from build123d import *

# Parameters (mm, degrees)
SKETCH1_R                    = 19.05
BOSS_EXTRUDE1_DEPTH          = 272.1102
SKETCH2_R                    = 12.7
CUT_EXTRUDE1_DEPTH           = 273.1102
F_1_1_4_7_TAPPED_HOLE1_D     = 28.17876
F_1_1_4_7_TAPPED_HOLE1_DEPTH = 49.022
F_1_1_4_7_TAPPED_HOLE1_TIP   = 8.465753589
F_1_1_4_7_TAPPED_HOLE2_D     = 28.17876
F_1_1_4_7_TAPPED_HOLE2_DEPTH = 49.022
F_1_1_4_7_TAPPED_HOLE2_TIP   = 8.465753589


with BuildPart() as part:
    # Sketch1 → Boss-Extrude1 (new body)
    with BuildSketch(Plane(origin=(0, 0, 0), x_dir=(1, 0, 0), z_dir=(0, 1, 0))):
        Circle(SKETCH1_R)
    extrude(amount=BOSS_EXTRUDE1_DEPTH)

    # Sketch2 → Cut-Extrude1 (cut, through all)
    with BuildSketch(Plane(origin=(0, 272.1102, 0), x_dir=(1, 0, 0), z_dir=(0, 1, 0))):
        Circle(SKETCH2_R)
    extrude(amount=-CUT_EXTRUDE1_DEPTH, mode=Mode.SUBTRACT)

    # 1-1/4-7 Tapped Hole1
    with Locations(Plane(origin=(0, 272.1102, 0), x_dir=(1, 0, 0), z_dir=(0, 1, 0))):
        with Locations((0, 0)):
            Hole(F_1_1_4_7_TAPPED_HOLE1_D / 2, depth=F_1_1_4_7_TAPPED_HOLE1_DEPTH)
            with Locations((0, 0, -(F_1_1_4_7_TAPPED_HOLE1_DEPTH + F_1_1_4_7_TAPPED_HOLE1_TIP / 2))):  # 118° drill point
                Cone(0, F_1_1_4_7_TAPPED_HOLE1_D / 2, F_1_1_4_7_TAPPED_HOLE1_TIP, mode=Mode.SUBTRACT)

    # 1-1/4-7 Tapped Hole2
    with Locations(Plane(origin=(0, 0, 0), x_dir=(-1, 0, 0), z_dir=(0, -1, 0))):
        with Locations((0, 0)):
            Hole(F_1_1_4_7_TAPPED_HOLE2_D / 2, depth=F_1_1_4_7_TAPPED_HOLE2_DEPTH)
            with Locations((0, 0, -(F_1_1_4_7_TAPPED_HOLE2_DEPTH + F_1_1_4_7_TAPPED_HOLE2_TIP / 2))):  # 118° drill point
                Cone(0, F_1_1_4_7_TAPPED_HOLE2_D / 2, F_1_1_4_7_TAPPED_HOLE2_TIP, mode=Mode.SUBTRACT)


solid = part.part
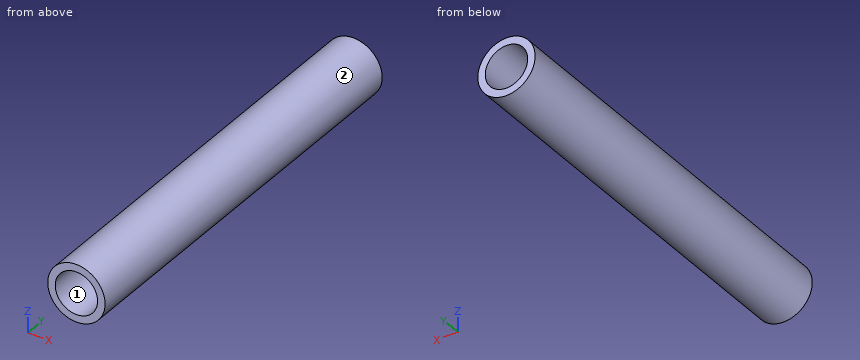
Check sheet for the modelled part. Datum: model origin and axes. Units: mm. Face numbers are marked on the shaded views. Coordinates: 2 decimals unless noted, no trailing zeros. Loops run counter-clockwise (first coordinate to the right, second up) from the corner with the lowest first, then second, coordinate; pieces in that order, holes last. Notation, with made-up numbers: (84, 64) -> (106, 64) arc R34 ccw to (106, 101) -> close; hole circle Ø8 at (-3.75, 82.5). An arc over 180 degrees is marked (long way). Write item = value, one per line. Start each with the question number.
1. Depth check by flat-ended pin: P1, Ø3, axis at x = 0.5, y = 67.5, coming from the -Z side; P2, Ø10, axis at x = -9.5, y = 99.5, coming from the -Z side; P3, Ø8, axis at x = -14.5, y = 162.5, coming from the -Z side; P4, Ø8, axis at x = 10, z = -13, coming from the -Y side. Enter the tip coordinate at first touch or a pass-through.
2. Material ranges on line 1 (Z direction, x = 0, y = 245.5); line 2 (X direction, y = 161, z = 0), recorded low to high.
3. Section check C-C on y = 201. Record the cut outline in (x, z).
4. Section check A-A on x = 0. Record the cut outline in (y, z).
5. Section check B-B on z = 0. Record the cut outline in (x, y), then the cut area to 3 significant figures.
6. Draft check along Z on the marked faces 1 and 2. Enter one of: released by +Z, released by -Z, zero draft, split by the parting line, or undercut.
Responses:
q1.P1 = -19.05
q1.P2 = -18.51
q1.P3 = -15.9
q1.P4 = 0
q2.line_1 = -19.05 to -14.09, 14.09 to 19.05
q2.line_2 = -19.05 to -12.7, 12.7 to 19.05
q3.outline = circle Ø38.1 at (0, 0); hole circle Ø25.4 at (0, 0)
q4.outline = (0, -19.05) -> (272.11, -19.05) -> (272.11, -14.09) -> (223.09, -14.09) -> (222.25, -12.7) -> (49.86, -12.7) -> (49.02, -14.09) -> (0, -14.09) -> close; (0, 14.09) -> (49.02, 14.09) -> (49.86, 12.7) -> (222.25, 12.7) -> (223.09, 14.09) -> (272.11, 14.09) -> (272.11, 19.05) -> (0, 19.05) -> close
q5.outline = (-19.05, 0) -> (-14.09, 0) -> (-14.09, 49.02) -> (-12.7, 49.86) -> (-12.7, 222.25) -> (-14.09, 223.09) -> (-14.09, 272.11) -> (-19.05, 272.11) -> close; (12.7, 49.86) -> (14.09, 49.02) -> (14.09, 0) -> (19.05, 0) -> (19.05, 272.11) -> (14.09, 272.11) -> (14.09, 223.09) -> (12.7, 222.25) -> close
q5.area = 3,180 mm2
q6.face_1 = undercut
q6.face_2 = split by the parting line
